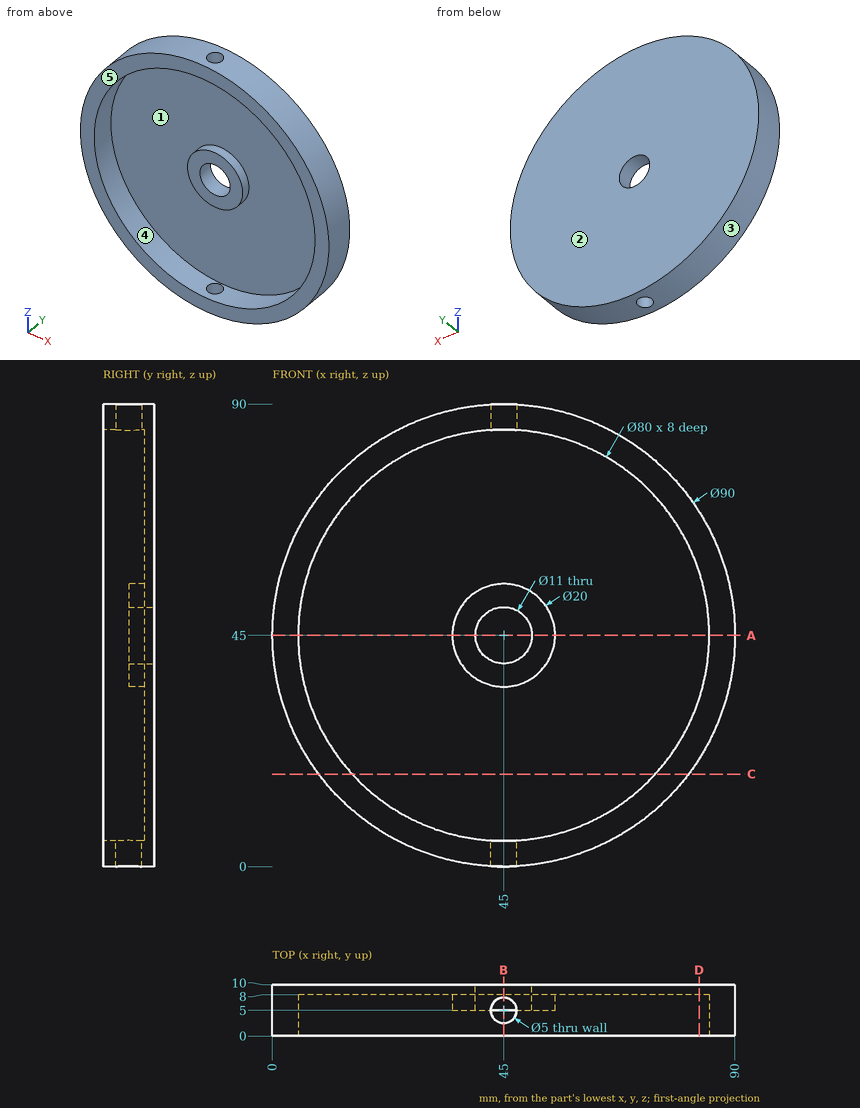
Part print with two shaded views. Sizes in mm from the minimum x, y, z corner. A direction names the side the tool comes from. Round coordinates to 2 decimals unless told otherwise and drop trailing zeros. Loops run counter-clockwise (first coordinate to the right, second up) from the corner with the lowest first, then second, coordinate; pieces in that order, holes last.
1. Slice it at B-B (x = 45). Give the cut face in (y, z), and give its area (3 significant figures).
Solutions:
outline: (0, 0) - (2.5, 0) - (2.5, 5) - (0, 5) - close; (0, 85) - (2.5, 85) - (2.5, 90) - (0, 90) - close; (5, 35) - (8, 35) - (8, 5) - (7.5, 5) - (7.5, 0) - (10, 0) - (10, 39.5) - (5, 39.5) - close; (5, 50.5) - (10, 50.5) - (10, 90) - (7.5, 90) - (7.5, 85) - (8, 85) - (8, 55) - (5, 55) - close
area: 215 mm2
2. Drill centre lines: line 1 along X through (y, z) = (7.25, 38); line 2 along Y through (x, z) = (44.5, 73); line 3 along Z through (x, y) = (47.5, 6). Where is each one in solid material? Low to high.
Solutions:
line 1: x = 0.55 to 5.62, 37.86 to 52.14, 84.38 to 89.45
line 2: y = 8 to 10
line 3: z = 0.07 to 5.08, 35.32 to 40.1, 49.9 to 54.68, 84.92 to 89.93
3. Two-plate mould, pull along X, no slides. Class the marked faces 3, 4 and 5: pulls with the +X half, pulls with the -X half, needs draft (parallel to the pull), parting line crosses it, or undercut.
Solutions:
face 3: parting line crosses it
face 4: undercut
face 5: needs draft
4. Slice it at A-A (z = 45). Give the cut face in (x, y), and give its area (3 significant figures).
Solutions:
outline: (0, 0) - (5, 0) - (5, 8) - (35, 8) - (35, 5) - (39.5, 5) - (39.5, 10) - (0, 10) - close; (50.5, 5) - (55, 5) - (55, 8) - (85, 8) - (85, 0) - (90, 0) - (90, 10) - (50.5, 10) - close
area: 265 mm2
5. Flat gauge pins, fed straight in: pin 1 (5 mm diameter, centred on x = 20.5, y = 7, fed in from +Z); pin 2 (1 mm diameter, centred on x = 14, z = 33.5, fed in from -Y); pin 3 (3 mm diameter, centred on y = 5, z = 61.5, fed in from -X). Where does each tip first touch, or does it go through?
Solutions:
pin 1: stops at z = 84.26
pin 2: stops at y = 8
pin 3: stops at x = 2.57
6. 3-axis set-ups, long thin cutter, end or side, ignore diameter. For the marked faces 1 and 2: which of +Z, -Z, +X, -X, +Y, -Y reach the whole face in a straight line?
Solutions:
face 1: -Y
face 2: +Z, -Z, +X, -X, +Y
7. Slice it at C-C (z = 18). Give the cut face in (x, y).
Solutions:
outline: (9, 0) - (15.49, 0) - (15.49, 8) - (74.51, 8) - (74.51, 0) - (81, 0) - (81, 10) - (9, 10) - close
8. Slice it at D-D (x = 83). Give the cut face in (y, z).
Solutions:
outline: (0, 20.9) - (10, 20.9) - (10, 69.1) - (0, 69.1) - (0, 57.49) - (8, 57.49) - (8, 32.51) - (0, 32.51) - close
